Part model, mm, in its own coordinate system. Face numbers are marked on the shaded views. A direction names the side the tool comes from. Coordinates: 2 decimals unless noted, no trailing zeros. Order: outer loops, then holes, each group sorted by start corner. A loop starts at its lowest first (then second) coordinate and runs counter-clockwise, first axis right, second up.
from build123d import *

# Parameters (mm, degrees)
SKETCH1_R               = 1.25
BOSS_EXTRUDE1_DEPTH     = 20
CUT_EXTRUDE1_DEPTH      = 30.021543722
CUT_EXTRUDE1_DEPTH_BACK = 30.021543722
SKETCH2_R               = 1.25
CUT_EXTRUDE2_DEPTH      = 29.565713714
CUT_EXTRUDE2_DEPTH_BACK = 29.565713714
SKETCH3_W               = 8
SKETCH3_H               = 4
FILLET1_R               = 2


with BuildPart() as part:
    # Sketch1 → Boss-Extrude1 (new body)
    with BuildSketch(Plane(origin=(0, 0, 0), x_dir=(1, 0, 0), z_dir=(0, 1, 0))):
        with BuildLine():
            Line((4, 0), (4, 20))
            Line((4, 20), (2.5, 20))
            Line((2.5, 20), (2.5, 15.120027663))
            Line((2.5, 15.120027663), (2.5, 6.5))
            ThreePointArc((2.5, 6.5), (1.767766953, 4.732233047), (0, 4))
            ThreePointArc((0, 4), (-2.828427125, -2.828427125), (4, 0))
        make_face()
        with Locations(Location((0, 0, 0), (0, 0, 270))):
            Circle(SKETCH1_R, mode=Mode.SUBTRACT)
    extrude(amount=BOSS_EXTRUDE1_DEPTH)

    # Sketch2 → Cut-Extrude1 (cut, two sides: drawn at the far end of the back side and taken through both)
    with BuildSketch(Plane.ZY.offset(-2.5).offset(-CUT_EXTRUDE1_DEPTH_BACK)):
        with Locations((-12.139236455, 10)):
            Circle(SKETCH2_R)
        with Locations((-15.86873762, 4)):
            Circle(SKETCH2_R)
        with Locations((-15.86873762, 16)):
            Circle(SKETCH2_R)
    extrude(amount=CUT_EXTRUDE1_DEPTH + CUT_EXTRUDE1_DEPTH_BACK, mode=Mode.SUBTRACT)

    # Sketch3 → Cut-Extrude2 (cut, two sides: drawn at the far end of the back side and taken through both)
    with BuildSketch(Plane(origin=(0, 0, 0), x_dir=(0, 0, -1), z_dir=(1, 0, 0)).offset(-CUT_EXTRUDE2_DEPTH_BACK)):
        with Locations((0, 10)):
            Rectangle(SKETCH3_W, SKETCH3_H)
    extrude(amount=CUT_EXTRUDE2_DEPTH + CUT_EXTRUDE2_DEPTH_BACK, mode=Mode.SUBTRACT)

    # Fillet1
    # the kernel refuses this fillet: 2 mm, written as the material it takes off along each edge
    with BuildSketch(Plane(origin=(2.5, -4.841229183, -20), x_dir=(0, 0, 1), z_dir=(0, 1, 0))) as fillet1_piece_1:
        with BuildLine():
            CenterArc((1.936491673, 2), FILLET1_R, 194.477512186, 75.522487814)
            Line((0, 1.5), (-0.038729833, 1.49))
            ThreePointArc((-0.038729833, 1.49), (-0.04, 0.75), (-0.04, 0))
            Line((-0.04, 0), (0, -0.04))
            Line((0, -0.04), (1.936491673, -0.04))
            Line((1.936491673, -0.04), (1.936491673, 0))
        make_face()
    extrude(amount=29.682458366, mode=Mode.SUBTRACT)
    with BuildSketch(Plane(origin=(0, 8, -4), x_dir=(0.7494414478105039, 0, -0.6620706278817206), z_dir=(0, 1, 0))) as fillet1_piece_2:
        with BuildLine():
            CenterArc((4.634494395, -1.498882896), FILLET1_R, 131.457982482, 83.620629792)
            Line((2.997765791, -2.648282512), (2.965031219, -2.671270504))
            ThreePointArc((2.965031219, -2.671270504), (1.472400071, -1.354118914), (-0.026482825, -0.029977658))
            Line((-0.026482825, -0.029977658), (0.026482825, 0.029977658))
            ThreePointArc((0.026482825, 0.029977658), (1.65517657, -0.58639638), (3.283870314, 0.029977658))
            Line((3.283870314, 0.029977658), (3.310353139, 0))
        make_face()
    extrude(amount=4, mode=Mode.SUBTRACT)


solid = part.part
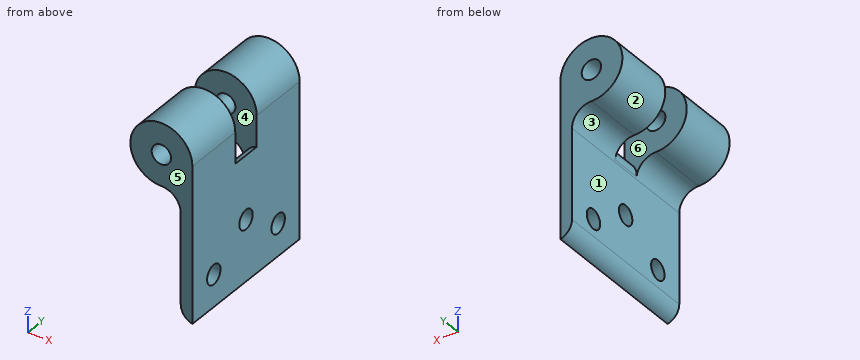
Q1. Mould opens along Y. For the marked faces 3, 4, 5 and 6 say: pulls with the +Y half, pulls with the -Y half, needs draft (parallel to the pull), parting line crosses it, or undercut.
Results list:
face 3: needs draft
face 4: undercut
face 5: pulls with the -Y half
face 6: undercut
Q2. Cut at C-C on y = 1.5. Write the cut outline in (x, z), and give its area (3 significant figures).
Results list:
outline: (0, -4) arc R2.5 cw to (2.5, -6.5) - (2.5, -18.06) arc R2 ccw to (4, -20) - (4, 0) arc R4 ccw (long way) to start; hole circle Ø2.5 at (0, 0)
area: 73.4 mm2
Q3. Wall check: line 1 along Z through (x, y) = (0, 6.25); line 2 along Y through (x, z) = (-1.5, -3.5); line 3 along Y through (x, z) = (3.25, -15). Give the ranges that are in metal, low to high.
Results list:
line 1: z = -4 to -1.25, 1.25 to 4
line 2: y = 0 to 8, 12 to 20
line 3: y = 0 to 3.1, 4.9 to 15.1, 16.9 to 20
Q4. Which spindle directions (+Z, -Z, +X, -X, +Y, -Y) get a long thin tool onto all of the face, cutting with end or side? Do the marked faces 1 and 2. Say none if no direction does.
Results list:
face 1: -Z, -X, +Y, -Y
face 2: +Y, -Y
Q5. Cut at D-D on y = 10. Write the cut outline in (x, z).
Results list:
outline: (2.48, -6.19) arc R2.5 cw to (2.5, -6.5) - (2.5, -10.89) - (4, -10.89) - (4, -4) arc R2 ccw to start; (2.5, -18.06) arc R2 ccw to (4, -20) - (4, -13.39) - (2.5, -13.39) - close
Q6. Cut at B-B on x = 2. Write the cut outline in (y, z), and give its area (3 significant figures).
Results list:
outline: (0, -5) - (8, -5) - (8, 3.46) - (0, 3.46) - close; (12, -5) - (20, -5) - (20, 3.46) - (12, 3.46) - close
area: 135 mm2
Q7. Pin check, flat tips, straight feed: pin 1 Ø1.5 at (x, y) = (3, 13.5) entering from -Z; pin 2 Ø6 at (y, z) = (8, -12) entering from -X; pin 3 Ø1.5 at (x, y) = (-1, 8.5) entering from -Z. Stop position of each tip, or through.
Results list:
pin 1: stops at z = -19.92
pin 2: stops at x = 2.5
pin 3: stops at z = -3.98
Q8. Cut at A-A on y = 4. Write the cut outline in (x, z), and give its area (3 significant figures).
Results list:
outline: (0, -4) arc R2.5 cw to (2.5, -6.5) - (2.5, -14.62) - (4, -14.62) - (4, 0) arc R4 ccw (long way) to start; (2.5, -18.06) arc R2 ccw to (4, -20) - (4, -17.12) - (2.5, -17.12) - close; hole circle Ø2.5 at (0, 0)
area: 69.6 mm2
